from build123d import *

# Parameters (mm, degrees)
F1_DEPTH = 25.4
F3_D     = 6.5278
F4_SIZE2 = 15.875
F4_SIZE  = 15.875
F5_R     = 5.08


with BuildPart() as f1:
    # F0 (on Top) → F1 (new body)
    with BuildSketch(Plane.XY):
        with BuildLine():
            Line((-65.826073072, 23.3069159811), (-65.826073072, 86.8069159811))
            Line((-65.826073072, 86.8069159811), (-68.366073072, 86.8069159811))
            Line((-68.366073072, 86.8069159811), (-68.366073072, 23.0399512236))
            Line((-68.366073072, 23.0399512236), (-52.5691465571, -51.2787448955))
            Line((-52.5691465571, -51.2787448955), (-52.5691465571, -218.829580138))
            ThreePointArc((-52.5691465571, -218.829580138), (-48.1054539024, -229.6058874832), (-37.3291465571, -234.069580138))
            Line((-37.3291465571, -234.069580138), (248.4208534429, -234.069580138))
            ThreePointArc((248.4208534429, -234.069580138), (259.1971607882, -229.6058874832), (263.6608534429, -218.829580138))
            Line((263.6608534429, -218.829580138), (263.6608534429, -51.2787448955))
            Line((263.6608534429, -51.2787448955), (279.4577799578, 23.0399512236))
            Line((279.4577799578, 23.0399512236), (279.4577799578, 86.8069159811))
            Line((279.4577799578, 86.8069159811), (276.9177799578, 86.8069159811))
            Line((276.9177799578, 86.8069159811), (276.9177799578, 23.3069159811))
            Line((276.9177799578, 23.3069159811), (261.1208534429, -51.011780138))
            Line((261.1208534429, -51.011780138), (261.1208534429, -218.829580138))
            ThreePointArc((261.1208534429, -218.829580138), (257.401109564, -227.809836259), (248.4208534429, -231.529580138))
            Line((248.4208534429, -231.529580138), (-37.3291465571, -231.529580138))
            ThreePointArc((-37.3291465571, -231.529580138), (-46.3094026781, -227.809836259), (-50.0291465571, -218.829580138))
            Line((-50.0291465571, -218.829580138), (-50.0291465571, -51.011780138))
            Line((-50.0291465571, -51.011780138), (-65.826073072, 23.3069159811))
        make_face()
    extrude(amount=F1_DEPTH)

    # F3 (through all)
    with Locations(Plane.YZ.offset(279.4577799578)):
        with Locations((58.0538512236, 12.7)):
            Hole(F3_D / 2)

    # F4
    f4_edges = [f1.edges().sort_by_distance(p)[0] for p in [
        (278.18778, 86.806916, 25.4),
        (-67.096073, 86.806916, 25.4),
    ]]
    chamfer(f4_edges, length=F4_SIZE, length2=F4_SIZE2)

    # F5
    f5_edges = [f1.edges().sort_by_distance(p)[0] for p in [
        (-67.096073, 70.931916, 25.4),
        (278.18778, 70.931916, 25.4),
        (278.18778, 86.806916, 9.525),
        (-67.096073, 86.806916, 9.525),
        (-67.096073, 86.806916, 0),
        (278.18778, 86.806916, 0),
    ]]
    fillet(f5_edges, radius=F5_R)


solid = f1.part
Verification items for the finished model (mm, model axes). A direction names the side the tool comes from. Give positions to 0.01 mm unless a question says otherwise; leave off trailing zeros. Loops run counter-clockwise (first coordinate to the right, second up) from the corner with the lowest first, then second, coordinate; pieces in that order, holes last.
1) Draft check along X on faces 4 (the flat face through (-67.08, 78.96, 17.37)), 5 (the flat face through (-50.029, -136, 13)), 6 (the flat face through (-52.569, -134, 13)). Enter one of: pulls with the +X half, pulls with the -X half, needs draft (parallel to the pull), parting line crosses it, or undercut.
2) Sectioned sample at B-B, the plane y = 1. Enter the section's corners in (x, z), then the cut area to 3 significant figures.
3) Sectioned sample at A-A, the plane y = -107. Enter the section's corners in (x, z), then the cut area to 3 significant figures.
4) Thickness scan on line 1 along X through (y, z) = (-75, 19); line 2 along Y through (x, z) = (-5.5, 19.5); line 3 along X through (y, z) = (13.5, 19). Record the ranges inside material, lowest first.
5) Sectioned sample at C-C, the plane x = 58.5. Enter the section's corners in (y, z).
6) Depth check by flat-ended pin: pin 1 Ø1.5 at (x, z) = (158, 13.5) entering from +Y; pin 2 Ø7.5 at (y, z) = (-156.5, 12) entering from +X; pin 3 Ø12.5 at (y, z) = (-101, 15.5) entering from -X; pin 4 Ø8.5 at (y, z) = (58.05, 12.7) entering from +X. Enter the tip coordinate at first touch or a pass-through.
7) Set-up check for faces 1 (the flat face through (104, -234.07, 13)), 2 (the flat face through (263.661, -136, 13)), 3 (the flat face through (-57.817, -14.373, 12.522)): record each of +Z, -Z, +X, -X, +Y, -Y from which the full face is reachable in a straight line by a thin tool's end or side.
Answers:
1. face 4: needs draft
1. face 5: undercut
1. face 6: pulls with the -X half
2. outline: (-63.68, 0) - (-61.08, 0) - (-61.08, 25.4) - (-63.68, 25.4) - close; (272.18, 0) - (274.77, 0) - (274.77, 25.4) - (272.18, 25.4) - close
2. area: 132 mm2
3. outline: (-52.57, 0) - (-50.03, 0) - (-50.03, 25.4) - (-52.57, 25.4) - close; (261.12, 0) - (263.66, 0) - (263.66, 25.4) - (261.12, 25.4) - close
3. area: 129 mm2
4. line 1: x = -52.57 to -50.03, 261.12 to 263.66
4. line 2: y = -234.07 to -231.53
4. line 3: x = -66.34 to -63.74, 274.83 to 277.43
5. outline: (-234.07, 0) - (-231.53, 0) - (-231.53, 25.4) - (-234.07, 25.4) - close
6. pin 1: stops at y = -231.53
6. pin 2: stops at x = 263.66
6. pin 3: stops at x = -52.57
6. pin 4: stops at x = 279.46
7. face 1: +Z, -Z, +X, -X, -Y
7. face 2: +Z, -Z, +X, -Y
7. face 3: +Z, -Z, +Y
